from build123d import *

# Parameters (mm, degrees)
SKETCH1_W           = 125
SKETCH1_H           = 65
BOSS_EXTRUDE1_DEPTH = 2
SKETCH2_W           = 125
SKETCH2_H           = 21.840489908
CUT_EXTRUDE1_DEPTH  = 3
CUT_EXTRUDE2_DEPTH  = 20
LPATTERN1_COUNT     = 9
LPATTERN1_PITCH     = 10


with BuildPart() as part:
    # Sketch1 → Boss-Extrude1 (new body)
    with BuildSketch(Plane.XY):
        Rectangle(SKETCH1_W, SKETCH1_H)
    extrude(amount=BOSS_EXTRUDE1_DEPTH)

    # Sketch2 → Cut-Extrude1 (cut, through all)
    with BuildSketch(Plane.XY.offset(2)):
        with Locations((0, 21.579755046)):
            Rectangle(SKETCH2_W, SKETCH2_H)
    extrude(amount=-CUT_EXTRUDE1_DEPTH, mode=Mode.SUBTRACT)

    # Sketch3 → Cut-Extrude2 (cut)
    with BuildSketch(Plane.XY.offset(2)):
        with BuildLine():
            Line((-45.774182217, -17.977174407), (-38.733037936, -1.547837751))
            ThreePointArc((-38.733037936, -1.547837751), (-37.046940168, -0.873398644), (-36.372501061, -2.559496412))
            Line((-36.372501061, -2.559496412), (-43.413645342, -18.988833068))
            ThreePointArc((-43.413645342, -18.988833068), (-45.09974311, -19.663272175), (-45.774182217, -17.977174407))
        make_face()
    cut_extrude2 = extrude(amount=-CUT_EXTRUDE2_DEPTH, mode=Mode.SUBTRACT)

    # LPattern1: Cut-Extrude2 ×9
    with Locations(*[(i * LPATTERN1_PITCH, 0, 0) for i in range(1, LPATTERN1_COUNT)]):
        add(cut_extrude2, mode=Mode.SUBTRACT)


solid = part.part
The listing builds one solid part. Answer for the finished solid, in the listing's coordinates (mm). Round coordinates to 2 decimals unless told otherwise and drop trailing zeros. Order: outer loops, then holes, each group sorted by start corner. A loop starts at its lowest first (then second) coordinate and runs counter-clockwise, first axis right, second up. Notation, with made-up numbers: (32, 12.5) -> (40, 12.5) arc R18 cw to (40, 40.5) -> close; hole circle Ø5 at (-15, 80). An arc over 180 degrees is marked (long way). Write each question's results on one line, items separated by ' | '. Start each with the question number.
Q1. The mould has two halves that part along Y. Classify faces 1 (the cylindrical face through (34.926, -19.674, 1.014)), 2 (the flat face through (27.697, -9.878, 1.014)): pulls with the +Y half, pulls with the -Y half, needs draft (parallel to the pull), parting line crosses it, or undercut.
Q2. Find section D-D (x = -2). Determine the outline of the cut face in (y, z), then the cut area to 3 significant figures.
Q3. Straight lines are drawn through the part: probe 1 along Y at (x, z) = (-30.5, 1.7); probe 2 along Y at (x, z) = (-23.5, 1.7). For each, find the intervals that lie inside material, in ascending order. Write a range as from..to.
Q4. Find section A-A (x = -44.5). Determine the outline of the cut face in (y, z).
Q5. Find section B-B (z = 0.7). Give the number of separate pieces and of enclosed holes in the cut face, then the cut area to 3 significant figures.
Worked answers:
1) face 1: undercut | face 2: undercut
2) outline: (-32.5, 0) -> (-15.69, 0) -> (-15.69, 2) -> (-32.5, 2) -> close; (-9.17, 0) -> (10.66, 0) -> (10.66, 2) -> (-9.17, 2) -> close | area: 73.3 mm2
3) probe 1: y = -32.5..-12.19, -5.67..10.66 | probe 2: y = -32.5..-19.16, -12.67..10.66
4) outline: (-32.5, 0) -> (-19.76, 0) -> (-19.76, 2) -> (-32.5, 2) -> close; (-15, 0) -> (10.66, 0) -> (10.66, 2) -> (-15, 2) -> close
5) separate pieces: 1 | enclosed holes: 9 | area: 4,940 mm2
